Can you work these out from the drawing? Everything is in mm from the part's minimum corner. A direction names the side the tool comes from. Give positions to 0.01 mm unless a question says otherwise; leave off trailing zeros. Write each loop counter-clockwise with the first axis right and the second up, starting at its lowest first coordinate (ties: lowest second). Pieces come first, ordered by that corner, then holes. Notation, with made-up numbers: M -7.5,79.25 L 40.5,79.25 A28 cw 40.5,113.25 Z; hole C -5,14.5 d5. An arc over 180 degrees is marked long. One line per item, written item: value.
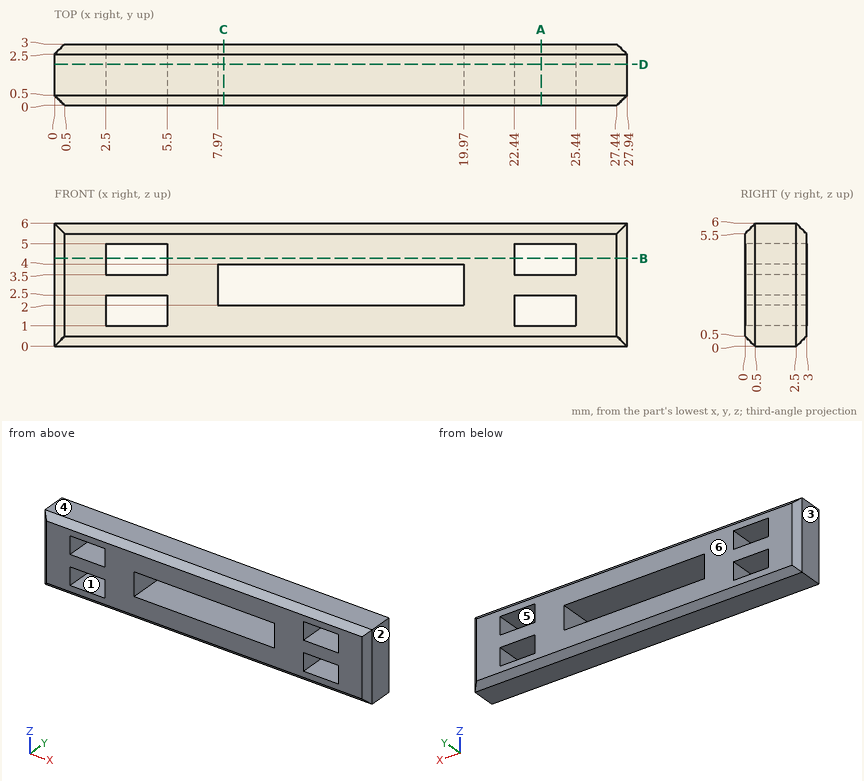
1) We'd pull the mould along X, two halves only. Please class the marked faces 1, 2, 3 and 4: pulls with the +X half, pulls with the -X half, needs draft (parallel to the pull), parting line crosses it, or undercut.
Outcome:
face 1: undercut
face 2: pulls with the +X half
face 3: pulls with the -X half
face 4: needs draft
2) On a 3-axis mill with a long thin cutter (end or side, diameter ignored), from which of +Z, -Z, +X, -X, +Y, -Y can I reach the whole of each face in a straight line? I mean the marked faces 5 and 6. Say none if no direction works.
Outcome:
face 5: +Y, -Y
face 6: +Z, -Z, +X, -X, +Y
3) If we section it at C-C, the plane x = 8.25: Write out the boundary of the cut face in (y, z).
Outcome:
outline: M 0,0.5 L 0.5,0 L 2.5,0 L 3,0.5 L 3,2 L 0,2 Z; M 0,4 L 3,4 L 3,5.5 L 2.5,6 L 0.5,6 L 0,5.5 Z
4) Please list where these lines run through material, in increasing order: L1, parallel to X at y = 0.7, z = 4.9; L2, parallel to Z at x = 24.5, y = 1.95; L3, parallel to X at y = 0.35, z = 2.1. Write a range as from..to.
Outcome:
L1: x = 0..2.5, 5.5..22.44, 25.44..27.94
L2: z = 0..1, 2.5..3.5, 5..6
L3: x = 0.15..2.5, 5.5..7.97, 19.97..22.44, 25.44..27.79
5) If we section it at B-B, the plane z = 4.3: Write out the boundary of the cut face in (x, y), then the cut area to 3 significant figures.
Outcome:
outline: M 0,0.5 L 0.5,0 L 2.5,0 L 2.5,3 L 0.5,3 L 0,2.5 Z; M 5.5,0 L 22.44,0 L 22.44,3 L 5.5,3 Z; M 25.44,0 L 27.44,0 L 27.94,0.5 L 27.94,2.5 L 27.44,3 L 25.44,3 Z
area: 65.3 mm^2
6) If we section it at A-A, the plane x = 23.75: Write out the boundary of the cut face in (y, z).
Outcome:
outline: M 0,0.5 L 0.5,0 L 2.5,0 L 3,0.5 L 3,1 L 0,1 Z; M 0,2.5 L 3,2.5 L 3,3.5 L 0,3.5 Z; M 0,5 L 3,5 L 3,5.5 L 2.5,6 L 0.5,6 L 0,5.5 Z
7) If we section it at D-D, the plane y = 2: Write out the boundary of the cut face in (x, z).
Outcome:
outline: M 0,0 L 27.94,0 L 27.94,6 L 0,6 Z; hole M 2.5,1 L 5.5,1 L 5.5,2.5 L 2.5,2.5 Z; hole M 2.5,3.5 L 5.5,3.5 L 5.5,5 L 2.5,5 Z; hole M 7.97,2 L 19.97,2 L 19.97,4 L 7.97,4 Z; hole M 22.44,1 L 25.44,1 L 25.44,2.5 L 22.44,2.5 Z; hole M 22.44,3.5 L 25.44,3.5 L 25.44,5 L 22.44,5 Z
